Job drawing, mm, ordinate dimensions from the low corner. One solid piece. A direction names the side the tool comes from. Round coordinates to 2 decimals unless told otherwise and drop trailing zeros. Loops run counter-clockwise (first coordinate to the right, second up) from the corner with the lowest first, then second, coordinate; pieces in that order, holes last. Notation, with made-up numbers: M 13.25,86 L 49.25,86 A15 cw 49.25,102 Z; hole C 78,37 d4. An arc over 180 degrees is marked long. Put each result on its own line as item: value. Start each with the question number.
1) Slice it at A-A on y = 7.75. Give the cut face in (x, z), then the cut area to 3 significant figures.
2) Drop flat-ended pins along their axis: pin 1 Ø1.5 at (x, z) = (3.5, 12) entering from -Y (1 decimal); pin 2 Ø3 at (y, z) = (7.5, 15) entering from -X; pin 3 Ø8 at (x, y) = (14.5, 5.5) entering from -Z; pin 4 Ø4 at (y, z) = (14.5, 18) entering from -X. Give the stop position or say it passes through.
3) Which spindle directions (+Z, -Z, +X, -X, +Y, -Y) get a long thin tool onto all of the face, cutting with end or side? Do the marked faces 1, 2 and 3. Say none if no direction does.
4) Slice it at D-D on z = 3.25. Give the cut face in (x, y) (1 decimal).
5) Probe line 1 along Y through (x, z) = (9.5, 3); line 2 along X through (y, z) = (9.5, 16.75) (1 decimal); line 3 along Z through (x, y) = (17.75, 10.25). List the from-to ranges inside material, lowest first.
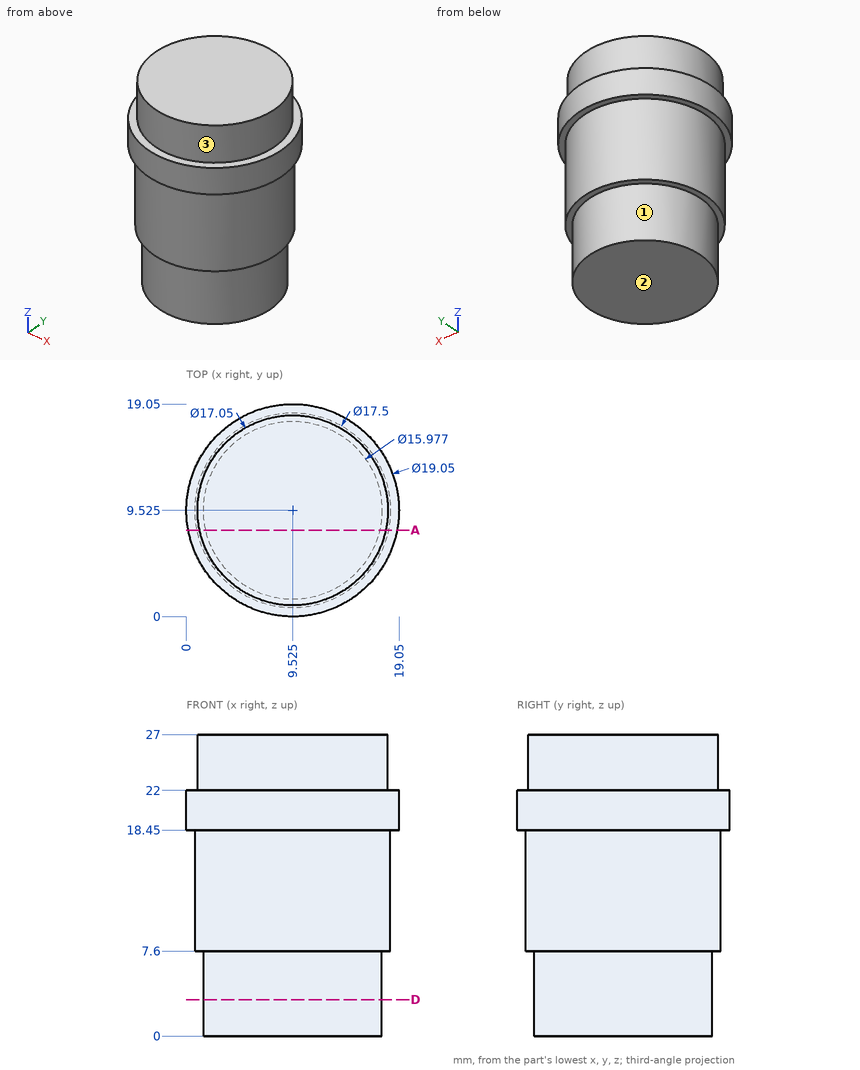
Recorded:
1. outline: M 0.17,18.45 L 0.96,18.45 L 0.96,7.6 L 1.74,7.6 L 1.74,0 L 17.31,0 L 17.31,7.6 L 18.09,7.6 L 18.09,18.45 L 18.88,18.45 L 18.88,22 L 17.86,22 L 17.86,27 L 1.19,27 L 1.19,22 L 0.17,22 Z
1. area: 454 mm2
2. pin 1: stops at y = 2.5
2. pin 2: stops at x = 0.79
2. pin 3: stops at z = 0
2. pin 4: stops at x = 0.49
3. face 1: -Z
3. face 2: -Z, +X, -X, +Y, -Y
3. face 3: +Z
4. outline: C 9.5,9.5 d16
5. line 1: y = 1.54 to 17.51
5. line 2: x = 0.8 to 18.3
5. line 3: z = 7.6 to 27
